Read the model definition and answer for the solid it produces. Units are mm, in the model's axes. Face numbers are marked on the shaded views. A direction names the side the tool comes from. Coordinates: 2 decimals unless noted, no trailing zeros. Write each loop counter-clockwise with the first axis right and the second up, starting at its lowest first coordinate (ties: lowest second). Pieces come first, ordered by that corner, then holes. Notation, with made-up numbers: (-3.5, 57) -> (46.5, 57) arc R13 ccw to (46.5, 65) -> close; hole circle Ø1 at (-27.5, -29.5). An arc over 180 degrees is marked (long way). Use CSV: the item, a comma, the result in double quotes.
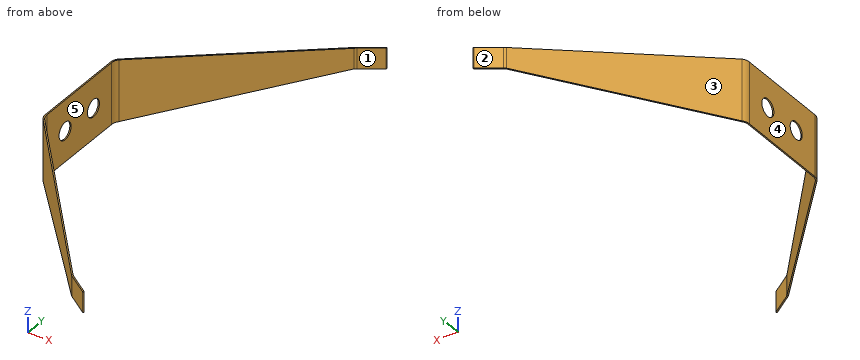
from build123d import *

# Parameters (mm, degrees)
ESTRUSIONE_ESTRUSIONE1_DEPTH      = 6
ESTRUSIONE_ESTRUSIONE1_DEPTH_BACK = 6
FORO_PER_VITE_M3_1_D              = 3.4
RACCORDO1_R                       = 2
RACCORDO2_R                       = 2
RACCORDO3_R                       = 2
RACCORDO4_R                       = 2
RACCORDO5_R                       = 2
RACCORDO6_R                       = 2
RACCORDO7_R                       = 2
RACCORDO8_R                       = 2
TAGLIO_ESTRUSIONE2_DEPTH          = 59.133547919
SCHIZZO6_W                        = 4
SCHIZZO6_H                        = 12.192194749
TAGLIO_ESTRUSIONE3_DEPTH          = 59.133547919


with BuildPart() as part:
    # Schizzo1 → Estrusione-Estrusione1 (new body, two sides)
    with BuildSketch(Plane.XY) as estrusione_estrusione1_sk:
        with BuildLine():
            Line((0, -10), (0, 10))
            Line((0, 10), (26.541757937, 40))
            Line((26.541757937, 40), (30.66238888, 42.832031185))
            ThreePointArc((30.66238888, 42.832031185), (30.836205433, 42.799816191), (30.803990439, 42.625999637))
            Line((30.803990439, 42.625999637), (26.708656989, 39.811354938))
            Line((26.708656989, 39.811354938), (0.25, 9.905283473))
            Line((0.25, 9.905283473), (0.25, -9.905283473))
            Line((0.25, -9.905283473), (26.708656989, -39.811354938))
            Line((26.708656989, -39.811354938), (30.803990439, -42.625999637))
            ThreePointArc((30.803990439, -42.625999637), (30.836205433, -42.799816191), (30.66238888, -42.832031185))
            Line((30.66238888, -42.832031185), (26.541757937, -40))
            Line((26.541757937, -40), (0, -10))
        make_face()
    extrude(amount=ESTRUSIONE_ESTRUSIONE1_DEPTH)
    extrude(estrusione_estrusione1_sk.sketch, amount=-ESTRUSIONE_ESTRUSIONE1_DEPTH_BACK)

    # Foro per Vite M3-1 (through all)
    with Locations(Plane(origin=(0.25, 0, 0), x_dir=(0, 0, -1), z_dir=(1, 0, 0))):
        with Locations((0, 4), (0, -4)):
            Hole(FORO_PER_VITE_M3_1_D / 2)

    # Raccordo1
    raccordo1_edges = [part.edges().sort_by_distance(p)[0] for p in [
        (0, 10, 0),
    ]]
    fillet(raccordo1_edges, radius=RACCORDO1_R)

    # Raccordo2
    raccordo2_edges = [part.edges().sort_by_distance(p)[0] for p in [
        (0, -10, 0),
    ]]
    fillet(raccordo2_edges, radius=RACCORDO2_R)

    # Raccordo3
    raccordo3_edges = [part.edges().sort_by_distance(p)[0] for p in [
        (26.541757937, -40, 0),
    ]]
    fillet(raccordo3_edges, radius=RACCORDO3_R)

    # Raccordo4
    raccordo4_edges = [part.edges().sort_by_distance(p)[0] for p in [
        (26.541757937, 40, 0),
    ]]
    fillet(raccordo4_edges, radius=RACCORDO4_R)

    # Raccordo5
    raccordo5_edges = [part.edges().sort_by_distance(p)[0] for p in [
        (0.25, -9.905283473, 0),
    ]]
    fillet(raccordo5_edges, radius=RACCORDO5_R)

    # Raccordo6
    raccordo6_edges = [part.edges().sort_by_distance(p)[0] for p in [
        (0.25, 9.905283473, 0),
    ]]
    fillet(raccordo6_edges, radius=RACCORDO6_R)

    # Raccordo7
    raccordo7_edges = [part.edges().sort_by_distance(p)[0] for p in [
        (26.708656989, 39.811354938, 0),
    ]]
    fillet(raccordo7_edges, radius=RACCORDO7_R)

    # Raccordo8
    raccordo8_edges = [part.edges().sort_by_distance(p)[0] for p in [
        (26.708656989, -39.811354938, 0),
    ]]
    fillet(raccordo8_edges, radius=RACCORDO8_R)

    # Schizzo4 → Taglio-Estrusione2 (cut, through all)
    with BuildSketch(Plane(origin=(-4.962730758, 4.390653283, 0), x_dir=(0, 0, 1), z_dir=(-0.748955721, 0.662620048, 0))):
        Polygon((2, 47.299760633), (6, 8.247289425), (6, 59.846735232), (2, 59.846735232), align=None)
        Polygon((-2, 47.299760633), (-6, 8.247289425), (-6, 59.846735232), (-2, 59.846735232), align=None)
    extrude(amount=-TAGLIO_ESTRUSIONE2_DEPTH, mode=Mode.SUBTRACT)

    # Schizzo6 → Taglio-Estrusione3 (cut, through all)
    with BuildSketch(Plane(origin=(-4.962730758, -4.390653283, 0), x_dir=(0, 0, 1), z_dir=(-0.748955721, -0.662620048, 0))):
        Polygon((-2, -47.299760633), (-6, -8.247289425), (-6, -47.299760633), align=None)
        with Locations((-4, -53.395858008)):
            Rectangle(SCHIZZO6_W, SCHIZZO6_H)
        with Locations((4, -53.395858008)):
            Rectangle(SCHIZZO6_W, SCHIZZO6_H)
        Polygon((6, -47.299760633), (6, -8.247289425), (2, -47.299760633), align=None)
    extrude(amount=-TAGLIO_ESTRUSIONE3_DEPTH, mode=Mode.SUBTRACT)


solid = part.part
1. A cutting plane is placed at A-A (z = 0). Give the number of separate pieces and of enclosed holes in the cut face, and give its area (3 significant figures).
Solutions:
separate pieces,"3"
enclosed holes,"0"
area,"25.8 mm^2"
2. For a pull along Y with two mould halves and no side action, classify the marked faces 3, 4 and 5 as pulls with the +Y half, pulls with the -Y half, needs draft (parallel to the pull), parting line crosses it, or undercut.
Solutions:
face 3,"pulls with the +Y half"
face 4,"needs draft"
face 5,"undercut"
3. A tool of negligible diameter and unlimited length cuts with its end or side. For the marked faces 1 and 2, from which of +Z, -Z, +X, -X, +Y, -Y can it reach the whole face along a straight path? Write none if from no direction.
Solutions:
face 1,"+Z, -Z, +X"
face 2,"+Z, -Z, -X, +Y"
4. A cutting plane is placed at C-C (x = 23). Give the vertices of the cut face in (y, z).
Solutions:
outline,"(-36, -2.52) -> (-35.62, -2.55) -> (-35.62, 2.55) -> (-36, 2.52) -> close; (35.62, -2.55) -> (36, -2.52) -> (36, 2.52) -> (35.62, 2.55) -> close"
5. Find the intervals of material crossed by line 1 along Y through (x, z) = (0.2, 0); line 2 along X through (y, z) = (4, 1.75); line 3 along Y through (x, z) = (2, -5.5), in increasing order.
Solutions:
line 1,"y = -10.11 to -5.7, -2.3 to 2.3, 5.7 to 10.11"
line 2,"x = 0 to 0.25"
line 3,"y = -12.26 to -11.88, 11.88 to 12.26"
6. Each of these flat-tipped pins is pushed along its axis until it touches: pin 1 Ø2.5 at (x, y) = (28, 42) entering from +Z; pin 2 Ø1 at (x, z) = (25.5, 0.5) entering from -Y; pin 3 Ø1.6 at (x, y) = (29, -42) entering from -Z; pin 4 Ø5 at (y, z) = (10.5, 3.5) entering from -X. Where does it stop, or does it pass through?
Solutions:
pin 1,"stops at z = 2"
pin 2,"stops at y = -39.39"
pin 3,"stops at z = -2"
pin 4,"stops at x = 0"
7. A cutting plane is placed at D-D (z = 4.75). Give the vertices of the cut face in (x, y).
Solutions:
outline,"(0, -9.24) arc R2 ccw to (0.5, -10.57) -> (8.59, -19.71) -> (8.78, -19.54) -> (0.75, -10.47) arc R2 cw to (0.25, -9.15) -> (0.25, 9.15) arc R2 cw to (0.75, 10.47) -> (8.78, 19.54) -> (8.59, 19.71) -> (0.5, 10.57) arc R2 ccw to (0, 9.24) -> close"
8. A cutting plane is placed at B-B (y = 4). Give the vertices of the cut face in (x, z), and give its area (3 significant figures).
Solutions:
outline,"(0, -6) -> (0.25, -6) -> (0.25, -1.7) -> (0, -1.7) -> close; (0, 1.7) -> (0.25, 1.7) -> (0.25, 6) -> (0, 6) -> close"
area,"2.15 mm^2"
